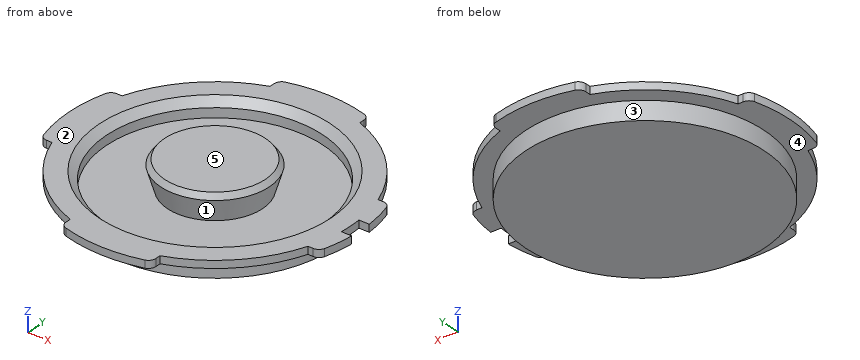
from build123d import *

# Parameters (mm, degrees)
CHAMFER001_SIZE           = 1.5
CYLINDER006_R             = 31
CYLINDER006_DEPTH         = 7
CHAMFER_SIZE              = 3
CYLINDER005_R             = 29
CYLINDER005_DEPTH         = 7
BOX004_W                  = 10
BOX004_H                  = 6
BOX004_DEPTH              = 10
BOX001_W                  = 100
BOX001_H                  = 40
BOX001_DEPTH              = 10
BOX_W                     = 100
BOX_H                     = 40
BOX_DEPTH                 = 10
CYLINDER003_R             = 39
CYLINDER003_DEPTH         = 2
FILLET_R                  = 2
FILLET001_R               = 2
BOX002_W                  = 100
BOX002_H                  = 40
BOX002_DEPTH              = 10
BOX003_W                  = 100
BOX003_H                  = 40
BOX003_DEPTH              = 10
CYLINDER004_R             = 39
CYLINDER004_DEPTH         = 2
FILLET003_R               = 2
FILLET002_R               = 2
FILLET002_PLACEMENT_ANGLE = 90
CYLINDER_R                = 32
CYLINDER_DEPTH            = 7
CYLINDER001_R             = 36.25
CYLINDER001_DEPTH         = 2


with BuildPart() as handle:
    # Cone → Cone (revolve)
    with BuildSketch(Plane.XZ):
        Polygon((0, 0), (12, 0), (15, 10), (0, 10), align=None)
    revolve(axis=Axis((0, 0, 0), (0, 0, 1)))

    # Chamfer001
    chamfer001_edges = [handle.edges().sort_by_distance(p)[0] for p in [
        (-15, 0, 10),
    ]]
    chamfer(chamfer001_edges, length=CHAMFER001_SIZE)


with BuildPart() as chamfer_body:
    # Cylinder006 → Cylinder006 (new body)
    with BuildSketch(Plane.XY.offset(4)):
        Circle(CYLINDER006_R)
    extrude(amount=CYLINDER006_DEPTH)

    # Chamfer
    chamfer_edges = [chamfer_body.edges().sort_by_distance(p)[0] for p in [
        (-31, 0, 4),
    ]]
    chamfer(chamfer_edges, length=CHAMFER_SIZE)


with BuildPart() as cylinder005:
    # Cylinder005 → Cylinder005 (new body)
    with BuildSketch(Plane.XY.offset(2.5)):
        Circle(CYLINDER005_R)
    extrude(amount=CYLINDER005_DEPTH)


with BuildPart() as cube004:
    # Box004 → Box004 (new body)
    with BuildSketch(Plane(origin=(36, -3, 0), x_dir=(1, 0, 0), z_dir=(0, 0, 1))):
        with Locations((5, 3)):
            Rectangle(BOX004_W, BOX004_H)
    extrude(amount=BOX004_DEPTH)


with BuildPart() as cube001:
    # Box001 → Box001 (new body)
    with BuildSketch(Plane(origin=(-50, -52, 0), x_dir=(1, 0, 0), z_dir=(0, 0, 1))):
        with Locations((50, 20)):
            Rectangle(BOX001_W, BOX001_H)
    extrude(amount=BOX001_DEPTH)


with BuildPart() as fusion:
    # Box → Box (new body)
    with BuildSketch(Plane(origin=(-50, 12, 0), x_dir=(1, 0, 0), z_dir=(0, 0, 1))):
        with Locations((50, 20)):
            Rectangle(BOX_W, BOX_H)
    extrude(amount=BOX_DEPTH)

    # Fusion: union Cube001
    add(cube001.part)


with BuildPart() as cut002:
    # Cylinder003 → Cylinder003 (new body)
    with BuildSketch(Plane.XY.offset(5)):
        Circle(CYLINDER003_R)
    extrude(amount=CYLINDER003_DEPTH)

    # Cut: cut Fusion
    add(fusion.part, mode=Mode.SUBTRACT)

    # Fillet
    fillet_edges = [cut002.edges().sort_by_distance(p)[0] for p in [
        (37.107951, -12, 6),
        (37.107951, 12, 6),
    ]]
    fillet(fillet_edges, radius=FILLET_R)

    # Fillet001
    fillet001_edges = [cut002.edges().sort_by_distance(p)[0] for p in [
        (-37.107951, -12, 6),
        (-37.107951, 12, 6),
    ]]
    fillet(fillet001_edges, radius=FILLET001_R)

    # Cut002: cut Cube004
    add(cube004.part, mode=Mode.SUBTRACT)


with BuildPart() as cube002:
    # Box002 → Box002 (new body)
    with BuildSketch(Plane(origin=(-50, -52, 0), x_dir=(1, 0, 0), z_dir=(0, 0, 1))):
        with Locations((50, 20)):
            Rectangle(BOX002_W, BOX002_H)
    extrude(amount=BOX002_DEPTH)


with BuildPart() as fusion001:
    # Box003 → Box003 (new body)
    with BuildSketch(Plane(origin=(-50, 12, 0), x_dir=(1, 0, 0), z_dir=(0, 0, 1))):
        with Locations((50, 20)):
            Rectangle(BOX003_W, BOX003_H)
    extrude(amount=BOX003_DEPTH)

    # Fusion001: union Cube002
    add(cube002.part)


with BuildPart() as bayonet:
    # Cylinder004 → Cylinder004 (new body)
    with BuildSketch(Plane.XY.offset(5)):
        Circle(CYLINDER004_R)
    extrude(amount=CYLINDER004_DEPTH)

    # Cut001: cut Fusion001
    add(fusion001.part, mode=Mode.SUBTRACT)

    # Fillet003
    fillet003_edges = [bayonet.edges().sort_by_distance(p)[0] for p in [
        (37.107951, -12, 6),
        (37.107951, 12, 6),
    ]]
    fillet(fillet003_edges, radius=FILLET003_R)

    # Fillet002
    fillet002_edges = [bayonet.edges().sort_by_distance(p)[0] for p in [
        (-37.107951, -12, 6),
        (-37.107951, 12, 6),
    ]]
    fillet(fillet002_edges, radius=FILLET002_R)


with BuildPart() as bayonet_1:
    # Fillet002 placement: moved
    add(bayonet.part.rotate(Axis((0, 0, 0), (0, 0, 1)), FILLET002_PLACEMENT_ANGLE))

    # Fusion002: union Cut002
    add(cut002.part)


with BuildPart() as fusion003:
    # Cylinder → Cylinder (new body)
    with BuildSketch(Plane.XY):
        Circle(CYLINDER_R)
    extrude(amount=CYLINDER_DEPTH)

    # Fusion003: union Bayonet
    add(bayonet_1.part)


with BuildPart() as oct19_body_port_cover:
    # Cylinder001 → Cylinder001 (new body)
    with BuildSketch(Plane.XY.offset(5)):
        Circle(CYLINDER001_R)
    extrude(amount=CYLINDER001_DEPTH)

    # Fusion004: union Fusion003
    add(fusion003.part)

    # Cut003: cut Cylinder005
    add(cylinder005.part, mode=Mode.SUBTRACT)

    # Cut004: cut Chamfer body
    add(chamfer_body.part, mode=Mode.SUBTRACT)

    # Fusion005: union Handle
    add(handle.part)


solid = oct19_body_port_cover.part
Input: part model. Units: mm. Frame: model coordinates. Face numbers are marked on the shaded views. A direction names the side the tool comes from. Give positions to 0.01 mm unless a question says otherwise; leave off trailing zeros. Loops run counter-clockwise (first coordinate to the right, second up) from the corner with the lowest first, then second, coordinate; pieces in that order, holes last. Notation, with made-up numbers: M 87,-34 L 126,-34 A9 ccw 126,-19 Z; hole C 14.25,55 d7. An arc over 180 degrees is marked long. Use one line per item in the form item = value.
1. First-contact query: pin 1 (3 mm diameter, centred on y = -1.5, z = 6, fed in from -X); pin 2 (5 mm diameter, centred on x = 2.5, y = -17, fed in from +Z); pin 3 (6 mm diameter, centred on x = -6.5, z = 4.5, fed in from +Y); pin 4 (2 mm diameter, centred on x = 21, y = -12.5, fed in from -Z). Flat tips, straight axial feed; report the tip coordinate or a pass-through.
Numbers:
pin_1 = -39
pin_2 = 2.5
pin_3 = 38.84
pin_4 = 0
2. Pull-direction query (Z, two-part tool) for the marked faces 1, 2 and 3; classes: released by +Z, released by -Z, zero draft, split by the parting line, or undercut.
Numbers:
face_1 = undercut
face_2 = released by +Z
face_3 = zero draft
3. Section query B-B, the plane y = 0. Return the cut outline in (x, z), and give its area (3 significant figures).
Numbers:
outline = M -39,5 L -32,5 L -32,0 L 32,0 L 32,5 L 36.25,5 L 36.25,7 L 31,7 L 29,5 L 29,2.5 L 12.75,2.5 L 14.57,8.56 L 13.5,10 L -13.5,10 L -14.57,8.56 L -12.75,2.5 L -29,2.5 L -29,5 L -31,7 L -39,7 Z
area = 411 mm²
4. Reachability of the marked faces 4 and 5 from +Z, -Z, +X, -X, +Y, -Y: full face, straight path, thin tool, end or side. Return the list, or none.
Numbers:
face_4 = -Z
face_5 = +Z, +X, -X, +Y, -Y
5. Section query A-A, the plane z = 6. Count the separate pieces of the cut face and the enclosed holes in it, and give its area (3 significant figures).
Numbers:
separate_pieces = 2
enclosed_holes = 1
area = 2,150 mm²
6. Line query: L1, parallel to X at y = -0.5, z = 5.25; L2, parallel to Y at x = 0, z = 4.45 (3 decimals); L3, parallel to Y at x = 0, z = 3.15 (3 decimals). Output: solid intervals per line, ascending.
Numbers:
L1 = -39 to -29.25, -13.57 to 13.57, 29.25 to 36.25
L2 = -32 to -29, -13.335 to 13.335, 29 to 32
L3 = -32 to -29, -12.945 to 12.945, 29 to 32
7. Section query C-C, the plane x = 0. Return the cut outline in (y, z), and give its area (3 significant figures).
Numbers:
outline = M -39,5 L -32,5 L -32,0 L 32,0 L 32,5 L 39,5 L 39,7 L 31,7 L 29,5 L 29,2.5 L 12.75,2.5 L 14.57,8.56 L 13.5,10 L -13.5,10 L -14.57,8.56 L -12.75,2.5 L -29,2.5 L -29,5 L -31,7 L -39,7 Z
area = 417 mm²
8. Section query D-D, the plane z = 1.25. Return the cut outline in (x, y), and give its area (3 significant figures).
Numbers:
outline = C 0,0 d64
area = 3,220 mm²
